Design review of the part built by this model. Coordinates are the model's own, in mm. A direction names the side the tool comes from. Give positions to 0.01 mm unless a question says otherwise; leave off trailing zeros. Write each loop counter-clockwise with the first axis right and the second up, starting at its lowest first coordinate (ties: lowest second). Pieces come first, ordered by that corner, then holes. Notation, with made-up numbers: M 11,56 L 16,56 A14 cw 16,75 Z; hole C 89.25,-38.5 d5. An arc over 180 degrees is marked long. Answer in a Markdown table with one row per item.
```python
from build123d import *

# Parameters (mm, degrees)
BOSS_EXTRUDE1_DEPTH      = 15
BOSS_EXTRUDE1_DEPTH_BACK = 15
SKETCH1_W                = 40
SKETCH1_H                = 25
SKETCH2_W                = 9
SKETCH2_H                = 6
SKETCH2_R                = 1.5
BOSS_EXTRUDE2_DEPTH      = 3
MIRROR3_COPY_1_SKETCH_W  = 9
MIRROR3_COPY_1_SKETCH_H  = 6
MIRROR3_COPY_1_SKETCH_R  = 1.5
MIRROR3_COPY_1_DEPTH     = 3
FILLET1_R                = 6


with BuildPart() as part:
    # Sketch1 → Boss-Extrude1 (new, two sides: drawn at the far end of the back side and taken through both)
    with BuildSketch(Plane.XY.offset(-BOSS_EXTRUDE1_DEPTH_BACK)):
        Rectangle(SKETCH1_W, SKETCH1_H)
        with BuildLine():
            Line((-8.4, 9.375), (8.4, 9.375))
            ThreePointArc((8.4, 9.375), (17.775, 0), (8.4, -9.375))
            Line((8.4, -9.375), (-8.4, -9.375))
            ThreePointArc((-8.4, -9.375), (-17.775, 0), (-8.4, 9.375))
        make_face(mode=Mode.SUBTRACT)
    extrude(amount=BOSS_EXTRUDE1_DEPTH + BOSS_EXTRUDE1_DEPTH_BACK)

    # Sketch2 → Boss-Extrude2 (add)
    with BuildSketch(Plane(origin=(20, 0, 0), x_dir=(0, 0, -1), z_dir=(1, 0, 0))):
        with Locations((-10.5, -15.5)):
            Rectangle(SKETCH2_W, SKETCH2_H)
        with Locations((-10.5, -15.5)):
            Circle(SKETCH2_R, mode=Mode.SUBTRACT)
    boss_extrude2 = extrude(amount=-BOSS_EXTRUDE2_DEPTH)

    # Mirror1: Boss-Extrude2 across plane
    add(boss_extrude2.mirror(Plane.XY))

    # Mirror3: Boss-Extrude2 across plane
    add(boss_extrude2.mirror(Plane(origin=(0, 0, 0), x_dir=(0, 0, 1), z_dir=(1, 0, 0))))

    # Mirror3 copy 1 sketch → Mirror3 copy 1 (add)
    with BuildSketch(Plane.ZY.offset(20)):
        with Locations((-10.5, -15.5)):
            Rectangle(MIRROR3_COPY_1_SKETCH_W, MIRROR3_COPY_1_SKETCH_H)
        with Locations((-10.5, -15.5)):
            Circle(MIRROR3_COPY_1_SKETCH_R, mode=Mode.SUBTRACT)
    extrude(amount=-MIRROR3_COPY_1_DEPTH)

    # Fillet1
    fillet1_edges = [part.edges().sort_by_distance(p)[0] for p in [
        (-18.5, -12.5, -6),
        (-18.5, -12.5, 6),
        (18.5, -12.5, -6),
        (18.5, -12.5, 6),
    ]]
    fillet(fillet1_edges, radius=FILLET1_R - 0.0001)  # a hair under: the kernel refuses the full size


solid = part.part
```
1) The part is to be moulded in two halves that separate along X. For faces 1 (the face through (0, -12.5, 0)), 2 (the face through (-20, -3, 0)), 3 (the face through (19, -18.5, 11)), say which applies: released by +X, released by -X, zero draft, split by the parting line, or undercut.
Geometry says:
| item | result |
|---|---|
| face 1 | undercut |
| face 2 | released by -X |
| face 3 | zero draft |
2) Add section B-B (x = 3.5). Write out the cut boundary in (y, z) (3 decimals), and give its area (4 significant figures).
Geometry says:
| item | result |
|---|---|
| outline | M -12.5,-15 L -9.375,-15 L -9.375,15 L -12.5,15 Z; M 9.375,-15 L 12.5,-15 L 12.5,15 L 9.375,15 Z |
| area | 187.5 mm^2 |
3) Add section C-C (z = 13). Write out the cut boundary in (x, y) (3 decimals).
Geometry says:
| item | result |
|---|---|
| outline | M -20,-18.5 L -17,-18.5 L -17,-12.5 L 17,-12.5 L 17,-18.5 L 20,-18.5 L 20,12.5 L -20,12.5 Z; hole M -8.4,-9.375 L 8.4,-9.375 A9.375 ccw 8.4,9.375 L -8.4,9.375 A9.375 ccw Z |
4) Insertion check: P1, Ø4, axis at x = -14.5, z = -5, coming from the -Y side; P2, Ø4, axis at y = -15.5, z = 10.5, coming from the +X side; P3, Ø8, axis at x = 2, y = -1.5, coming from the -Z side (3 decimals). Each pin has a flat end and moves straight along its axis. Give the tip position at first contact, or say it passes through.
Geometry says:
| item | result |
|---|---|
| P1 | y = -12.5 |
| P2 | x = 20 |
| P3 | through |
5) Add section A-A (y = 0). Write out the cut boundary in (x, z) (3 decimals).
Geometry says:
| item | result |
|---|---|
| outline | M -20,-15 L -17.775,-15 L -17.775,15 L -20,15 Z; M 17.775,-15 L 20,-15 L 20,15 L 17.775,15 Z |
6) Add section D-D (y = -15). Count the separate pieces of the cut face and the enclosed holes in it, and give its area (3 significant figures).
Geometry says:
| item | result |
|---|---|
| separate pieces | 8 |
| enclosed holes | 0 |
| area | 87.6 mm^2 |
7) To check wall thickness, follow probe 1 along Y at (x, z) = (-6, 13.5) (3 decimals); probe 2 along Y at (x, z) = (18.75, -10.5); probe 3 along X at (y, z) = (-13.5, 13.25). State the ranges of each line that lie inside material, in increasing order. Write a range as [from, to].
Geometry says:
| item | result |
|---|---|
| probe 1 | [-12.5, -9.375], [9.375, 12.5] |
| probe 2 | [-18.5, -17], [-14, 12.5] |
| probe 3 | [-20, -17], [17, 20] |
8) For faces 4 (the face through (-17, -14, 9)), 5 (the face through (-18.52, -15.43, 12)), 6 (the face through (17.773, 0.206, -0.21)), 7 (the face through (-19, -18.5, 11)), 8 (the face through (18.479, -14.304, -4.289)), list the 3-axis set-ups (+Z, -Z, +X, -X, +Y, -Y) from which the entire face can be reached by the end or side of a thin tool; tool diameter is ignored.
Geometry says:
| item | result |
|---|---|
| face 4 | +Z, -Z, -Y |
| face 5 | +X, -X |
| face 6 | +Z, -Z |
| face 7 | +Z, -Z, +X, -X, -Y |
| face 8 | +X, -X, -Y |
